from build123d import *

# Parameters (mm, degrees)
SKETCH1_R            = 0.5
BOSS_EXTRUDE1_DEPTH  = 0.7
FILLET1_R            = 1
FILLET2_R            = 0.5
BOSS_EXTRUDE2_DEPTH  = 5.1
SKETCH3_R            = 2.25
BOSS_EXTRUDE7_DEPTH  = 6
SKETCH4_W            = 5
SKETCH4_H            = 5
BOSS_EXTRUDE8_DEPTH  = 1
SKETCH5_R            = 3.5
BOSS_EXTRUDE9_DEPTH  = 2
SKETCH6_W            = 2.7
SKETCH6_H            = 1
BOSS_EXTRUDE10_DEPTH = 6
FILLET3_R            = 1


with BuildPart() as part:
    # Sketch1 → Boss-Extrude1 (new body)
    with BuildSketch(Plane(origin=(0, 0, 0), x_dir=(1, 0, 0), z_dir=(0, 1, 0))):
        Polygon((0, 0), (2.94, 0), (2.94, 2.025), (15.34, 2.025), (15.34, 0), (18.24, 0), (18.24, 2.025), (17.62, 2.025), (17.62, 12.825), (18.24, 12.825), (18.24, 14.85), (15.34, 14.85), (15.34, 12.825), (2.94, 12.825), (2.94, 14.85), (0, 14.85), (0, 12.825), (0.62, 12.825), (0.62, 2.025), (0, 2.025), align=None)
        with Locations(Location((1.5, 13.325, 0), (0, 0, 270))):
            Circle(SKETCH1_R, mode=Mode.SUBTRACT)
        with Locations(Location((1.5, 1.525, 0), (0, 0, 270))):
            Circle(SKETCH1_R, mode=Mode.SUBTRACT)
        with Locations(Location((16.74, 1.525, 0), (0, 0, 270))):
            Circle(SKETCH1_R, mode=Mode.SUBTRACT)
        with Locations(Location((16.74, 13.325, 0), (0, 0, 270))):
            Circle(SKETCH1_R, mode=Mode.SUBTRACT)
    extrude(amount=BOSS_EXTRUDE1_DEPTH)

    # Fillet1
    fillet1_edges = [part.edges().sort_by_distance(p)[0] for p in [
        (2.94, 0.35, -12.825),
        (15.34, 0.35, -12.825),
        (15.34, 0.35, -2.025),
        (2.94, 0.35, -2.025),
    ]]
    fillet(fillet1_edges, radius=FILLET1_R)

    # Fillet2
    fillet2_edges = [part.edges().sort_by_distance(p)[0] for p in [
        (0, 0.35, -2.025),
        (0.62, 0.35, -12.825),
        (0, 0.35, -14.85),
        (2.94, 0.35, -14.85),
        (15.34, 0.35, -14.85),
        (18.24, 0.35, -14.85),
        (17.62, 0.35, -12.825),
        (17.62, 0.35, -2.025),
        (18.24, 0.35, 0),
        (15.34, 0.35, 0),
        (2.94, 0.35, 0),
        (0, 0.35, 0),
    ]]
    fillet(fillet2_edges, radius=FILLET2_R)

    # Sketch2 → Boss-Extrude2 (add)
    with BuildSketch(Plane(origin=(0, 0.7, 0), x_dir=(1, 0, 0), z_dir=(0, 1, 0))):
        Polygon((0.62, 2.725), (16.62, 2.725), (16.62, 7.425), (8.62, 7.425), (8.62, 12.125), (0.62, 12.125), align=None)
    extrude(amount=BOSS_EXTRUDE2_DEPTH)

    # Sketch3 → Boss-Extrude7 (add)
    with BuildSketch(Plane(origin=(8.62, 0, 0), x_dir=(0, 0, -1), z_dir=(1, 0, 0))):
        with Locations(Location((9.775, 3.25, 0), (0, 0, 180))):
            Circle(SKETCH3_R)
    extrude(amount=BOSS_EXTRUDE7_DEPTH)

    # Sketch4 → Boss-Extrude8 (add)
    with BuildSketch(Plane.XZ):
        with Locations((9.14, -7.175)):
            Rectangle(SKETCH4_W, SKETCH4_H)
    extrude(amount=BOSS_EXTRUDE8_DEPTH)

    # Sketch5 → Boss-Extrude9 (add)
    with BuildSketch(Plane.ZY.offset(-0.62)):
        with Locations(Location((-4.95, 2.9, 0), (0, 0, 124.04773237))):
            Circle(SKETCH5_R)
    extrude(amount=BOSS_EXTRUDE9_DEPTH)

    # Sketch6 → Boss-Extrude10 (add)
    with BuildSketch(Plane(origin=(0, 5.8, 0), x_dir=(1, 0, 0), z_dir=(0, 1, 0))):
        with Locations((7.27, 5.075)):
            Rectangle(SKETCH6_W, SKETCH6_H)
    extrude(amount=BOSS_EXTRUDE10_DEPTH)

    # Fillet3
    fillet3_edges = [part.edges().sort_by_distance(p)[0] for p in [
        (5.92, 11.8, -5.075),
        (8.62, 11.8, -5.075),
    ]]
    fillet(fillet3_edges, radius=FILLET3_R)


solid = part.part
Work out the finished part from the listing and answer in its coordinate system (mm). A direction names the side the tool comes from. Round coordinates to 2 decimals unless told otherwise and drop trailing zeros. Loops run counter-clockwise (first coordinate to the right, second up) from the corner with the lowest first, then second, coordinate; pieces in that order, holes last. Notation, with made-up numbers: (28, 11.25) -> (56, 11.25) arc R25 ccw to (56, 46.25) -> close; hole circle Ø2 at (64, 81.25). An arc over 180 degrees is marked (long way). Use one line per item in the form item = value.
(1) Find section C-C on x = 9.75. Give the vertices of the cut face in (y, z) (3 decimals).
Answer list:
outline = (-1, -9.675) -> (0, -9.675) -> (0, -12.825) -> (0.7, -12.825) -> (0.7, -7.425) -> (5.8, -7.425) -> (5.8, -2.725) -> (0.7, -2.725) -> (0.7, -2.025) -> (0, -2.025) -> (0, -4.675) -> (-1, -4.675) -> close; circle Ø4.5 at (3.25, -9.775)
(2) Straight lines are drawn through the part: line 1 (X direction, y = 0.5, z = -5.5); line 2 (Y direction, x = 4.5, z = -9.75); line 3 (Z direction, x = 5.25, y = 4.5) (3 decimals). For each, find the intervals that lie inside material, in ascending order.
Answer list:
line_1 = -1.38 to 17.62
line_2 = 0 to 5.8
line_3 = -12.125 to -2.725
(3) A tool of negligible diameter and unlimited length cuts with its end or side. For faces 4 (the flat face through (16.62, 3, -5)), 5 (the flat face through (0.62, 3, -2)), 6 (the flat face through (5, 3, -12.125)), 7 (the cylindrical face through (3.225, 0.355, -13.126)), from which of +Z, -Z, +X, -X, +Y, -Y can it reach the whole face along a straight path? Write none if from no direction.
Answer list:
face_4 = +Z, -Z, +X, +Y
face_5 = +Z, +X, +Y
face_6 = -Z, +X, -X, +Y
face_7 = -Z, +Y, -Y
(4) Find section A-A on x = 1.5. Give the vertices of the cut face in (y, z) (3 decimals), then the cut area to 3 significant figures.
Answer list:
outline = (0, -14.85) -> (0.7, -14.85) -> (0.7, -13.825) -> (0, -13.825) -> close; (0, -12.825) -> (0.7, -12.825) -> (0.7, -12.125) -> (5.8, -12.125) -> (5.8, -2.725) -> (0.7, -2.725) -> (0.7, -2.025) -> (0, -2.025) -> close; (0, -1.025) -> (0.7, -1.025) -> (0.7, 0) -> (0, 0) -> close
area = 56.9 mm2
(5) Flat-ended cylindrical pins translate along their axes: P1, Ø1.5, axis at x = 13, z = -13, coming from the +Y side; P2, Ø1.5, axis at x = 7, z = -3.5, coming from the -Y side; P3, Ø0.8, axis at y = -0.5, z = -8.5, coming from the -X side; P4, Ø1, axis at x = 2, y = 7.5, coming from the +Z side. Find the tip coordinate at first contact, or state that the pin passes through.
Answer list:
P1 = 0.7
P2 = 0
P3 = 6.64
P4 = through
(6) For a pull along Z with two mould halves and no side action, classify faces 1 (the cylindrical face through (1.84, 0.35, -1.89)), 2 (the flat face through (7, 9, -4.575)), 3 (the cylindrical face through (6.205, 11.499, -5.082)) as released by +Z, released by -Z, zero draft, split by the parting line, or undercut.
Answer list:
face_1 = undercut
face_2 = released by +Z
face_3 = zero draft
(7) Find section B-B on z = -4.95. Give the vertices of the cut face in (x, y).
Answer list:
outline = (-1.38, -0.6) -> (0.62, -0.6) -> (0.62, 0) -> (6.64, 0) -> (6.64, -1) -> (11.64, -1) -> (11.64, 0) -> (17.62, 0) -> (17.62, 0.7) -> (16.62, 0.7) -> (16.62, 5.8) -> (8.62, 5.8) -> (8.62, 10.8) arc R1 ccw to (7.62, 11.8) -> (6.92, 11.8) arc R1 ccw to (5.92, 10.8) -> (5.92, 5.8) -> (0.62, 5.8) -> (0.62, 6.4) -> (-1.38, 6.4) -> close
(8) Find section D-D on y = 2.9. Give the vertices of the cut face in (x, z) (3 decimals), then the cut area to 3 significant figures.
Answer list:
outline = (-1.38, -8.45) -> (0.62, -8.45) -> (0.62, -12.125) -> (8.62, -12.125) -> (8.62, -11.998) -> (14.62, -11.998) -> (14.62, -7.552) -> (8.62, -7.552) -> (8.62, -7.425) -> (16.62, -7.425) -> (16.62, -2.725) -> (0.62, -2.725) -> (0.62, -1.45) -> (-1.38, -1.45) -> close
area = 153 mm2
